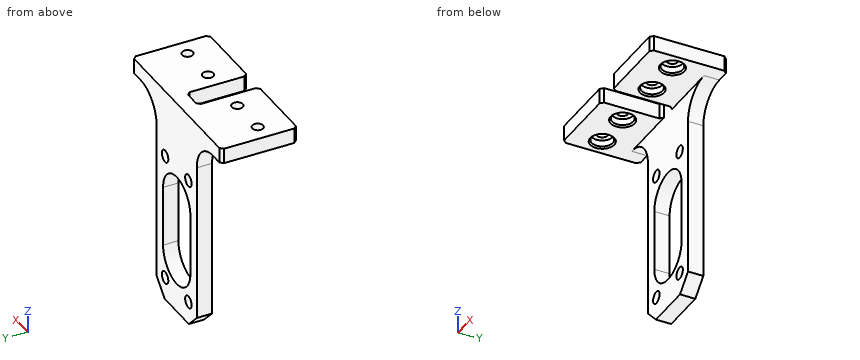
from build123d import *

# Parameters (mm, degrees)
SKETCH1_W           = 25
SKETCH1_H           = 72
SKETCH1_W_2         = 15
SKETCH1_H_2         = 5
BOSS_EXTRUDE1_DEPTH = 5
SKETCH2_R           = 2
CUT_EXTRUDE1_DEPTH  = 46.576858163
CHAMFER1_SIZE       = 5
CUT_EXTRUDE2_DEPTH  = 46.576858163
SKETCH5_W           = 24
SKETCH5_H           = 5
BOSS_EXTRUDE3_DEPTH = 20
FILLET2_R           = 10
CHAMFER3_SIZE       = 1
HOLE1_D             = 3.556
HOLE1_CBORE_D       = 6.858
HOLE1_CBORE_DEPTH   = 2.54
CHAMFER4_SIZE       = 0.5


with BuildPart() as part:
    # Sketch1 → Boss-Extrude1 (new body)
    with BuildSketch(Plane(origin=(0, 0, 0), x_dir=(1, 0, 0), z_dir=(0, 1, 0))):
        Rectangle(SKETCH1_W, SKETCH1_H)
        with Locations((-20, -33.5)):
            Rectangle(SKETCH1_W_2, SKETCH1_H_2)
        with Locations((20, -33.5)):
            Rectangle(SKETCH1_W_2, SKETCH1_H_2)
    extrude(amount=BOSS_EXTRUDE1_DEPTH)

    # Sketch2 → Cut-Extrude1 (cut, through all)
    with BuildSketch(Plane(origin=(0, 5, 0), x_dir=(1, 0, 0), z_dir=(0, 1, 0))):
        with Locations(Location((-7.25, 28.5, 0), (0, 0, 270))):
            Circle(SKETCH2_R)
        with Locations(Location((7.25, 28.5, 0), (0, 0, 270))):
            Circle(SKETCH2_R)
        with Locations(Location((-7.25, -13.5, 0), (0, 0, 270))):
            Circle(SKETCH2_R)
        with Locations(Location((7.25, -13.5, 0), (0, 0, 270))):
            Circle(SKETCH2_R)
    extrude(amount=-CUT_EXTRUDE1_DEPTH, mode=Mode.SUBTRACT)

    # Chamfer1
    chamfer1_edges = [part.edges().sort_by_distance(p)[0] for p in [
        (-12.5, 2.5, -36),
        (12.5, 2.5, -36),
    ]]
    chamfer(chamfer1_edges, length=CHAMFER1_SIZE)

    # Sketch3 → Cut-Extrude2 (cut, through all)
    with BuildSketch(Plane(origin=(0, 5, 0), x_dir=(1, 0, 0), z_dir=(0, 1, 0))):
        with BuildLine():
            Line((-8.5, -2), (-8.5, 18))
            ThreePointArc((-8.5, 18), (0, 26.5), (8.5, 18))
            Line((8.5, 18), (8.5, -2))
            ThreePointArc((8.5, -2), (0, -10.5), (-8.5, -2))
        make_face()
    extrude(amount=-CUT_EXTRUDE2_DEPTH, mode=Mode.SUBTRACT)

    # Sketch5 → Boss-Extrude3 (add)
    with BuildSketch(Plane(origin=(0, 0, 0), x_dir=(-1, 0, 0), z_dir=(0, -1, 0))):
        with Locations((15.5, -33.5)):
            Rectangle(SKETCH5_W, SKETCH5_H)
        with Locations((-15.5, -33.5)):
            Rectangle(SKETCH5_W, SKETCH5_H)
    extrude(amount=BOSS_EXTRUDE3_DEPTH)

    # Fillet2
    fillet2_edges = [part.edges().sort_by_distance(p)[0] for p in [
        (-12.5, 2.5, 31),
        (12.5, 2.5, 31),
    ]]
    fillet(fillet2_edges, radius=FILLET2_R)

    # Chamfer3
    chamfer3_edges = [part.edges().sort_by_distance(p)[0] for p in [
        (27.5, 5, 33.5),
        (-27.5, 5, 33.5),
        (-3.5, 0, 33.5),
        (-27.5, -20, 33.5),
        (-3.5, -20, 33.5),
        (3.5, 0, 33.5),
        (27.5, -20, 33.5),
        (3.5, -20, 33.5),
    ]]
    chamfer(chamfer3_edges, length=CHAMFER3_SIZE)

    # Hole1 (through all)
    with Locations(Plane(origin=(0, 0, 31), x_dir=(-1, 0, 0), z_dir=(0, 0, -1))):
        with Locations((-21.85, -10), (-9.15, -10), (9.15, -10), (21.85, -10)):
            CounterBoreHole(HOLE1_D / 2, HOLE1_CBORE_D / 2, HOLE1_CBORE_DEPTH)

    # Chamfer4
    chamfer4_edges = [part.edges().sort_by_distance(p)[0] for p in [
        (-18.421, -10, 31),
        (-5.721, -10, 31),
        (12.579, -10, 31),
        (25.279, -10, 31),
    ]]
    chamfer(chamfer4_edges, length=CHAMFER4_SIZE)


solid = part.part
Build history of the part. All positions in model axes, mm. Round coordinates to 2 decimals unless told otherwise and drop trailing zeros. Loops run counter-clockwise (first coordinate to the right, second up) from the corner with the lowest first, then second, coordinate; pieces in that order, holes last. Notation, with made-up numbers: (31.5, 9.5) -> (49.5, 9.5) arc R26 cw to (49.5, 23.5) -> close; hole circle Ø7 at (-19.75, -2.5). An arc over 180 degrees is marked (long way). Answer in a Markdown table with one row per item.
Item 1: Pin check, flat tips, straight feed: pin 1 (12 mm diameter, centred on y = -13, z = 19.5, fed in from -X) (3 decimals); pin 2 (4 mm diameter, centred on y = 3, z = -10.5, fed in from +X); pin 3 (12 mm diameter, centred on x = -22, y = -0.5, fed in from -Z); pin 4 (5.5 mm diameter, centred on x = -10, y = -10, fed in from -Z). Stop position of each tip, or through.
Answers below:
| item | result |
|---|---|
| pin 1 | passes through |
| pin 2 | stops at x = 12.5 |
| pin 3 | stops at z = 28.62 |
| pin 4 | stops at z = 31.33 |
Item 2: Saw through at B-B (x = 0). Write the cut outline in (y, z).
Answers below:
| item | result |
|---|---|
| outline | (0, -36) -> (5, -36) -> (5, -26.5) -> (0, -26.5) -> close; (0, 10.5) -> (5, 10.5) -> (5, 36) -> (0, 36) -> close |
Item 3: Saw through at C-C (z = 18.5). Write the cut outline in (x, y).
Answers below:
| item | result |
|---|---|
| outline | (-12.5, 0) -> (12.5, 0) -> (12.5, 5) -> (-12.5, 5) -> close |
Item 4: Saw through at A-A (z = -22). Write the cut outline in (x, y), and give its area (3 significant figures).
Answers below:
| item | result |
|---|---|
| outline | (-12.5, 0) -> (-7.5, 0) -> (-7.5, 5) -> (-12.5, 5) -> close; (7.5, 0) -> (12.5, 0) -> (12.5, 5) -> (7.5, 5) -> close |
| area | 50.0 mm² |
Item 5: Drill centre lines: L1, parallel to X at y = 2.7, z = -28.5; L2, parallel to Y at x = 9.15, z = 34.55; L3, parallel to X at y = 3, z = -18. Where is each one in solid material? Low to high. Write a range as [from, to].
Answers below:
| item | result |
|---|---|
| L1 | x = [-12.5, -9.25], [-5.25, 5.25], [9.25, 12.5] |
| L2 | y = [-20, -11.78], [-8.22, 5] |
| L3 | x = [-12.5, -8.5], [8.5, 12.5] |
